Geometry: final body of the model. Coordinates: model frame, mm. A direction names the side the tool comes from. Give positions to 0.01 mm unless a question says otherwise; leave off trailing zeros. Order: outer loops, then holes, each group sorted by start corner. A loop starts at its lowest first (then second) coordinate and runs counter-clockwise, first axis right, second up. Notation, with made-up numbers: (82.5, 88.5) - (103.5, 88.5) arc R31 cw to (103.5, 115.5) - close; hole circle Ø4 at (73, 82). An arc over 180 degrees is marked (long way). One line per item, written item: value.
```python
from build123d import *

# Parameters (mm, degrees)
SKETCH_1_W          = 30
SKETCH_1_H          = 3
SKETCH_1_W_2        = 8
SKETCH_1_H_2        = 2.2
EXTRUDE_2_DEPTH     = 2.5
SKETCH_2_R          = 1.65
CUT_EXTRUDE_1_DEPTH = 14
SKETCH_3_W          = 5
SKETCH_3_H          = 2.8
CUT_EXTRUDE_2_DEPTH = 14
SKETCH_5_R          = 1.6
CUT_EXTRUDE_3_DEPTH = 50


with BuildPart() as part:
    # 草图1 → 凸台-拉伸2 (new, symmetric)
    with BuildSketch(Plane.XY):
        with Locations((0, 2.6)):
            Rectangle(SKETCH_1_W, SKETCH_1_H)
        with Locations((-11, 0)):
            Rectangle(SKETCH_1_W_2, SKETCH_1_H_2)
        with Locations((0, -2.6)):
            Rectangle(SKETCH_1_W, SKETCH_1_H)
    extrude(amount=EXTRUDE_2_DEPTH, both=True)

    # 草图2 → 切除-拉伸1 (cut)
    with BuildSketch(Plane.XY.offset(2.5)):
        with Locations((-11, 0)):
            Circle(SKETCH_2_R)
    extrude(amount=-CUT_EXTRUDE_1_DEPTH, mode=Mode.SUBTRACT)

    # 草图3 → 切除-拉伸2 (cut)
    with BuildSketch(Plane.XY.offset(2.5)):
        with Locations((4, 0)):
            Rectangle(SKETCH_3_W, SKETCH_3_H)
    extrude(amount=-CUT_EXTRUDE_2_DEPTH, mode=Mode.SUBTRACT)

    # 草图5 → 切除-拉伸3 (cut)
    with BuildSketch(Plane(origin=(0, 4.1, 0), x_dir=(1, 0, 0), z_dir=(0, 1, 0))):
        with Locations(Location((11, 0, 0), (0, 0, 180))):
            Circle(SKETCH_5_R)
    extrude(amount=-CUT_EXTRUDE_3_DEPTH, mode=Mode.SUBTRACT)


solid = part.part
```
1) Mould query, pull axis Z, two halves, no side actions, for faces 4 (the face through (0, 2, 2.5)), 5 (the face through (15, -3, 0)), 6 (the face through (12.6, 2.62, 0.07)), 7 (the face through (12.6, -2.58, 0.07)). Classes: released by +Z, released by -Z, zero draft, split by the parting line, or undercut.
Answers below:
face 4: released by +Z
face 5: zero draft
face 6: undercut
face 7: undercut
2) First-contact query: pin 1 (1.1 mm diameter, centred on y = 0, z = -1, fed in from +X); pin 2 (1 mm diameter, centred on x = 6.5, y = -0.5, fed in from +Z). Flat tips, straight axial feed; report the tip coordinate or a pass-through.
Answers below:
pin 1: x = -7
pin 2: through
3) Material intervals for line 1 along Y through (x, z) = (0, 1.15); line 2 along Z through (x, y) = (11, 2.95); line 3 along Y through (x, z) = (-11, 0.95), sorted ascending.
Answers below:
line 1: -4.1 to -1.1, 1.1 to 4.1
line 2: -2.5 to -1.6, 1.6 to 2.5
line 3: -4.1 to -1.65, 1.65 to 4.1
4) Section B-B, the plane x = 5. Return loops of the section in (y, z), then the cut area to 3 significant figures.
Answers below:
outline: (-4.1, -2.5) - (-1.4, -2.5) - (-1.4, 2.5) - (-4.1, 2.5) - close; (1.4, -2.5) - (4.1, -2.5) - (4.1, 2.5) - (1.4, 2.5) - close
area: 27.0 mm^2
5) Set-up query: faces 1 (the face through (4, -1.4, 0)), 2 (the face through (0, -4.1, 0)), 3 (the face through (-3, 1.1, 0)). Return all of +Z, -Z, +X, -X, +Y, -Y with unobstructed straight access to the full face (end or side cutting, diameter ignored); none if empty.
Answers below:
face 1: +Z, -Z
face 2: +Z, -Z, +X, -X, -Y
face 3: +Z, -Z, +X
6) Section C-C, the plane y = 0. Return loops of the section in (x, z).
Answers below:
outline: (-15, -2.5) - (-12.65, -2.5) - (-12.65, 2.5) - (-15, 2.5) - close; (-9.35, -2.5) - (-7, -2.5) - (-7, 2.5) - (-9.35, 2.5) - close
7) Section A-A, the plane z = 0. Return loops of the section in (x, y).
Answers below:
outline: (-15, -4.1) - (9.4, -4.1) - (9.4, -1.1) - (6.5, -1.1) - (6.5, -1.4) - (1.5, -1.4) - (1.5, -1.1) - (-7, -1.1) - (-7, 1.1) - (1.5, 1.1) - (1.5, 1.4) - (6.5, 1.4) - (6.5, 1.1) - (9.4, 1.1) - (9.4, 4.1) - (-15, 4.1) - close; (12.6, -4.1) - (15, -4.1) - (15, -1.1) - (12.6, -1.1) - close; (12.6, 1.1) - (15, 1.1) - (15, 4.1) - (12.6, 4.1) - close; hole circle Ø3.3 at (-11, 0)
8) Section D-D, the plane x = 11. Return loops of the section in (y, z), then the cut area to 3 significant figures.
Answers below:
outline: (-4.1, -2.5) - (-1.1, -2.5) - (-1.1, -1.6) - (-4.1, -1.6) - close; (-4.1, 1.6) - (-1.1, 1.6) - (-1.1, 2.5) - (-4.1, 2.5) - close; (1.1, -2.5) - (4.1, -2.5) - (4.1, -1.6) - (1.1, -1.6) - close; (1.1, 1.6) - (4.1, 1.6) - (4.1, 2.5) - (1.1, 2.5) - close
area: 10.8 mm^2
